Design review of the part built by this model. Coordinates are the model's own, in mm. Coordinates: 2 decimals unless noted, no trailing zeros. Write each loop counter-clockwise with the first axis right and the second up, starting at its lowest first coordinate (ties: lowest second). Pieces come first, ordered by that corner, then holes.
Q1. Take a section at B-B, the plane x = -3.5. Write out the cut boundary in (y, z), plus the area to 3 significant figures.
Q2. For pin 1 Ø1.5 at (y, z) = (-7, 9) entering from +X; pin 2 Ø4 at (x, y) = (30, -3) entering from +Z; pin 3 Ø4 at (y, z) = (-2.5, 10.5) entering from +X, all flat-tipped, find the tip position at first contact; note any pin that passes through.
Q3. For L1, parallel to Z at x = -4, y = -6.5; L2, parallel to Z at x = 2, y = -7; L3, parallel to X at y = -3, z = 15, list the stretches that pass through material, from the lowest coordinate up.
Q4. Take a section at A-A, the plane y = -2.5. Write out the cut boundary in (x, z).
Q5. Take a section at C-C, the plane z = 0. Write out the cut boundary in (x, y), plus the area to 3 significant figures.
from build123d import *

# Parameters (mm, degrees)
BOSS_EXTRUDE1_DEPTH = 8
BOSS_EXTRUDE1_DRAFT = -35


with BuildPart() as part:
    # Sketch1 → Boss-Extrude1 (with draft: the straight prism first)
    with BuildSketch(Plane(origin=(0, 0, 0), x_dir=(1, 0, 0), z_dir=(0, 1, 0))):
        with BuildLine():
            ThreePointArc((-34.5, 26.25), (-42.278174593, 23.028174593), (-45.5, 15.25))
            Line((-45.5, 15.25), (-45.5, -15.25))
            ThreePointArc((-45.5, -15.25), (-42.278174593, -23.028174593), (-34.5, -26.25))
            Line((-34.5, -26.25), (34.5, -26.25))
            ThreePointArc((34.5, -26.25), (42.278174593, -23.028174593), (45.5, -15.25))
            Line((45.5, -15.25), (45.5, 15.25))
            ThreePointArc((45.5, 15.25), (42.278174593, 23.028174593), (34.5, 26.25))
            Line((34.5, 26.25), (-34.5, 26.25))
        make_face()
    extrude(amount=-BOSS_EXTRUDE1_DEPTH)
    # Boss-Extrude1: the draft: its side faces are tilted about the plane it starts from
    boss_extrude1_sides = [part.faces().sort_by_distance(p)[0] for p in [
        (-42.278174593, -4, -23.028174593),
        (-45.5, -4, 0),
        (-42.278174593, -4, 23.028174593),
        (0, -4, 26.25),
        (42.278174593, -4, 23.028174593),
        (45.5, -4, 0),
        (42.278174593, -4, -23.028174593),
        (0, -4, -26.25),
    ]]
    draft(boss_extrude1_sides, Plane(origin=(0, 0, 0), x_dir=(1, 0, 0), z_dir=(0, 1, 0)), BOSS_EXTRUDE1_DRAFT)


solid = part.part
Responses:
1. outline: (-8, -20.65) - (0, -26.25) - (0, 26.25) - (-8, 20.65) - close
1. area: 375 mm2
2. pin 1: stops at x = 41.12
2. pin 2: stops at z = 25.55
2. pin 3: stops at x = 45.15
3. L1: z = -21.7 to 21.7
3. L2: z = -21.35 to 21.35
3. L3: x = -43.4 to 43.4
4. outline: (-43.75, -15.25) arc R9.25 ccw to (-34.5, -24.5) - (34.5, -24.5) arc R9.25 ccw to (43.75, -15.25) - (43.75, 15.25) arc R9.25 ccw to (34.5, 24.5) - (-34.5, 24.5) arc R9.25 ccw to (-43.75, 15.25) - close
5. outline: (-45.5, 0) - (-39.9, -8) - (39.9, -8) - (45.5, 0) - close
5. area: 683 mm2
